```python
from build123d import *

# Parameters (mm, degrees)
BASPROSKE_W         = 15
BASPROSKE_H         = 12
TOOTHCUT_DEPTH      = 23.649503306
TEETHCUTS_COUNT     = 10
TEETHCUTS_ANGLE     = 324
BORSKE_R            = 0.45
BORE_DEPTH          = 50.0000508
SKETCH1_R           = 0.45
CUT_EXTRUDE1_DEPTH  = 15
SKETCH2_R           = 3.991106517
BOSS_EXTRUDE1_DEPTH = 15
SKETCH3_R           = 35
BOSS_EXTRUDE2_DEPTH = 5
SKETCH7_R           = 1.6
CUT_EXTRUDE2_DEPTH  = 10
CUT_EXTRUDE3_DEPTH  = 3
CUT_EXTRUDE5_DEPTH  = 3


with BuildPart() as part:
    # BasProSke → Base-Revolve (revolve)
    with BuildSketch(Plane(origin=(0, 0, 0), x_dir=(1, 0, 0), z_dir=(0, 1, 0)), mode=Mode.PRIVATE) as base_revolve_sk:
        with Locations((7.5, 6)):
            Rectangle(BASPROSKE_W, BASPROSKE_H)
    revolve(base_revolve_sk.sketch.rotate(Axis((-10, 0, 0), (1, 0, 0)), 180), axis=Axis((-10, 0, 0), (1, 0, 0)))

    # TooCutSke → ToothCut (cut, through all)
    with BuildSketch(Plane(origin=(0, 0, 0), x_dir=(0, 0, -1), z_dir=(1, 0, 0))):
        with BuildLine():
            ThreePointArc((1.173662691, 7.406586048), (0, 7.499), (-1.173662691, 7.406586048))
            ThreePointArc((-1.173662691, 7.406586048), (-1.668191438, 9.834565786), (-3.497907776, 11.50542856))
            ThreePointArc((-3.497907776, 11.50542856), (0, 12.0254), (3.497907776, 11.50542856))
            ThreePointArc((3.497907776, 11.50542856), (1.668191438, 9.834565786), (1.173662691, 7.406586048))
        make_face()
    toothcut = extrude(amount=TOOTHCUT_DEPTH, mode=Mode.SUBTRACT)

    # TeethCuts: ToothCut ×10 about axis
    teethcuts_axis = Axis((-10, 0, 0), (1, 0, 0))
    for i in range(1, TEETHCUTS_COUNT):
        add(toothcut.rotate(teethcuts_axis, i * TEETHCUTS_ANGLE / (TEETHCUTS_COUNT - 1)), mode=Mode.SUBTRACT)

    # BorSke → Bore (cut, symmetric)
    with BuildSketch(Plane(origin=(0, 0, 0), x_dir=(0, 0, -1), z_dir=(1, 0, 0))):
        with Locations(Location((0, 0, 0), (0, 0, 180))):
            Circle(BORSKE_R)
    extrude(amount=BORE_DEPTH, both=True, mode=Mode.SUBTRACT)

    # Sketch1 → Cut-Extrude1 (cut)
    with BuildSketch(Plane.ZY):
        with BuildLine():
            Line((1.212435565, 2.3), (-1.212435565, 2.3))
            ThreePointArc((-1.212435565, 2.3), (-1.343068786, -2.226244873), (2.6, 0))
            ThreePointArc((2.6, 0), (2.226244873, 1.343068786), (1.212435565, 2.3))
        make_face()
        Circle(SKETCH1_R, mode=Mode.SUBTRACT)
    extrude(amount=-CUT_EXTRUDE1_DEPTH, mode=Mode.SUBTRACT)

    # Sketch2 → Boss-Extrude1 (add)
    with BuildSketch(Plane.ZY):
        Circle(SKETCH2_R)
    extrude(amount=-BOSS_EXTRUDE1_DEPTH)

    # Sketch3 → Boss-Extrude2 (add)
    with BuildSketch(Plane.ZY):
        Circle(SKETCH3_R)
    extrude(amount=BOSS_EXTRUDE2_DEPTH)

    # Sketch7 → Cut-Extrude2 (cut)
    with BuildSketch(Plane.ZY.offset(5)):
        with Locations((30, 0)):
            Circle(SKETCH7_R)
        with Locations((-15, -25.980762114)):
            Circle(SKETCH7_R)
        with Locations((-15, 25.980762114)):
            Circle(SKETCH7_R)
    extrude(amount=-CUT_EXTRUDE2_DEPTH, mode=Mode.SUBTRACT)

    # Sketch8 → Cut-Extrude3 (cut)
    with BuildSketch(Plane(origin=(0, 0, 0), x_dir=(0, 0, -1), z_dir=(1, 0, 0))):
        Polygon((15.808290377, 27.380762114), (14.191709623, 27.380762114), (13.383419246, 25.980762114), (14.191709623, 24.580762114), (15.808290377, 24.580762114), (16.616580754, 25.980762114), align=None)
        Polygon((-31.616580754, 0), (-30.808290377, -1.4), (-29.191709623, -1.4), (-28.383419246, 0), (-29.191709623, 1.4), (-30.808290377, 1.4), align=None)
        Polygon((15.808290377, -27.380762114), (16.616580754, -25.980762114), (15.808290377, -24.580762114), (14.191709623, -24.580762114), (13.383419246, -25.980762114), (14.191709623, -27.380762114), align=None)
    extrude(amount=-CUT_EXTRUDE3_DEPTH, mode=Mode.SUBTRACT)

    # Sketch9 → Cut-Extrude5 (cut)
    with BuildSketch(Plane(origin=(0, 0, 0), x_dir=(0, 0, -1), z_dir=(1, 0, 0))):
        Polygon((16.616580754, 28.780762114), (13.383419246, 28.780762114), (11.766838493, 25.980762114), (13.383419246, 23.180762114), (16.616580754, 23.180762114), (18.233161507, 25.980762114), align=None)
        Polygon((-33.233161507, 0), (-31.616580754, -2.8), (-28.383419246, -2.8), (-26.766838493, 0), (-28.383419246, 2.8), (-31.616580754, 2.8), align=None)
        Polygon((16.616580754, -28.780762114), (18.233161507, -25.980762114), (16.616580754, -23.180762114), (13.383419246, -23.180762114), (11.766838493, -25.980762114), (13.383419246, -28.780762114), align=None)
    extrude(amount=-CUT_EXTRUDE5_DEPTH, mode=Mode.SUBTRACT)


solid = part.part
```
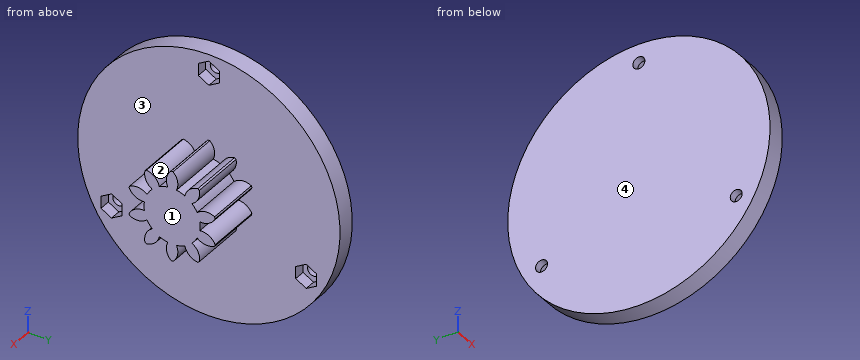
Part model, mm, in its own coordinate system. Face numbers are marked on the shaded views. A direction names the side the tool comes from. Round coordinates to 2 decimals unless told otherwise and drop trailing zeros. Write each loop counter-clockwise with the first axis right and the second up, starting at its lowest first coordinate (ties: lowest second). Pieces come first, ordered by that corner, then holes.
Item 1: Cut at A-A, the plane x = -1. Give the cut face in (y, z).
Results:
outline: circle Ø70 at (0, 0); hole (-28.78, -16.62) - (-25.98, -18.23) - (-23.18, -16.62) - (-23.18, -13.38) - (-25.98, -11.77) - (-28.78, -13.38) - close; hole (-2.8, 28.38) - (0, 26.77) - (2.8, 28.38) - (2.8, 31.62) - (0, 33.23) - (-2.8, 31.62) - close; hole (23.18, -16.62) - (25.98, -18.23) - (28.78, -16.62) - (28.78, -13.38) - (25.98, -11.77) - (23.18, -13.38) - close
Item 2: Two-plate mould, pull along Y, no slides. Class the marked faces 1 and 2: +Y half, -Y half, draft (parallel to the pull), parting line (faces both ways), or undercut.
Results:
face 1: draft
face 2: undercut
Item 3: Probe L1, parallel to Y at x = 10, z = -4; L2, parallel to Y at x = -3.6, z = -15; L3, parallel to X at y = -23.5, z = 18. List the from-to ranges inside material, lowest first.
Results:
L1: y = -11.24 to -7.53, -6.34 to 6.34, 7.53 to 11.24
L2: y = -31.62 to -27.58, -24.38 to 24.38, 27.58 to 31.62
L3: x = -5 to 0
Item 4: Cut at B-B, the plane z = 30. Give the cut face in (x, y).
Results:
outline: (-5, -18.03) - (0, -18.03) - (0, -2.8) - (-3, -2.8) - (-3, -1.6) - (-5, -1.6) - close; (-5, 1.6) - (-3, 1.6) - (-3, 2.8) - (0, 2.8) - (0, 18.03) - (-5, 18.03) - close
Item 5: Drop flat-ended pins along their axis: pin 1 Ø2.5 at (x, z) = (-1.5, 29.5) entering from -Y; pin 2 Ø1.5 at (x, z) = (-2, -14.5) entering from +Y; pin 3 Ø3 at (x, z) = (-0.5, -26) entering from -Y (3 decimals). Give the stop position or say it passes through.
Results:
pin 1: stops at y = -20.66
pin 2: stops at y = 32.19
pin 3: stops at y = -24.995
Item 6: Cut at D-D, the plane y = -9.5. Give the cut face in (x, z).
Results:
outline: (-5, -33.69) - (0, -33.69) - (0, -4.45) - (15, -4.45) - (15, -1.5) - (0, -1.5) - (0, 1.5) - (15, 1.5) - (15, 4.45) - (0, 4.45) - (0, 33.69) - (-5, 33.69) - close
Item 7: Cut at C-C, the plane z = 0. Give the cut face in (x, y).
Results:
outline: (-5, -35) - (0, -35) - (0, -7.5) - (15, -7.5) - (15, 7.5) - (0, 7.5) - (0, 35) - (-5, 35) - close
Item 8: Which spindle directions (+Z, -Z, +X, -X, +Y, -Y) get a long thin tool onto all of the face, cutting with end or side? Do the marked faces 3 and 4. Say none if no direction does.
Results:
face 3: +X
face 4: +Z, -Z, -X, +Y, -Y
